Verification items for the finished model (mm, model axes). Round coordinates to 2 decimals unless told otherwise and drop trailing zeros. Order: outer loops, then holes, each group sorted by start corner. A loop starts at its lowest first (then second) coordinate and runs counter-clockwise, first axis right, second up. Notation, with made-up numbers: (7, 4.5) -> (46, 4.5) arc R25 cw to (46, 37.5) -> close; hole circle Ø5 at (32.25, 84). An arc over 180 degrees is marked (long way). Put each result on its own line as item: value.
from build123d import *

# Parameters (mm, degrees)
SKETCH1_W           = 100
SKETCH1_H           = 11.7
BOSS_EXTRUDE1_DEPTH = 2.85
SKETCH2_R           = 1.75
CUT_EXTRUDE3_DEPTH  = 51.421671928
SKETCH3_R           = 2.4
CUT_EXTRUDE4_DEPTH  = 51.662732852


with BuildPart() as part:
    # Sketch1 → Boss-Extrude1 (new body)
    with BuildSketch(Plane(origin=(0, 0, 0), x_dir=(1, 0, 0), z_dir=(0, 1, 0))):
        Rectangle(SKETCH1_W, SKETCH1_H)
    extrude(amount=BOSS_EXTRUDE1_DEPTH)

    # Sketch2 → Cut-Extrude3 (cut, through all)
    with BuildSketch(Plane(origin=(0, 2.85, 0), x_dir=(1, 0, 0), z_dir=(0, 1, 0))):
        with Locations(Location((0, 0, 0), (0, 0, 270))):
            Circle(SKETCH2_R)
    extrude(amount=-CUT_EXTRUDE3_DEPTH, mode=Mode.SUBTRACT)

    # Sketch3 → Cut-Extrude4 (cut, through all)
    with BuildSketch(Plane.XZ.offset(2.85)):
        with Locations(Location((-37.5, 0, 0), (0, 0, 270))):
            Circle(SKETCH3_R)
        with Locations(Location((37.5, 0, 0), (0, 0, 270))):
            Circle(SKETCH3_R)
    extrude(amount=-CUT_EXTRUDE4_DEPTH, mode=Mode.SUBTRACT)


solid = part.part
Item 1: Material ranges on L1, parallel to X at y = 1.7, z = 0; L2, parallel to X at y = 1.9, z = 2; L3, parallel to X at y = 1.55, z = 0.5, recorded low to high. Write a range as [from, to].
Check sheet entries:
L1: x = [-50, -39.9], [-35.1, -1.75], [1.75, 35.1], [39.9, 50]
L2: x = [-50, -38.83], [-36.17, 36.17], [38.83, 50]
L3: x = [-50, -39.85], [-35.15, -1.68], [1.68, 35.15], [39.85, 50]
Item 2: Section check B-B on y = 0.9. Record the boundary of the cut face in (x, z), then the cut area to 3 significant figures.
Check sheet entries:
outline: (-50, -5.85) -> (50, -5.85) -> (50, 5.85) -> (-50, 5.85) -> close; hole circle Ø4.8 at (-37.5, 0); hole circle Ø3.5 at (0, 0); hole circle Ø4.8 at (37.5, 0)
area: 1,120 mm^2
Item 3: Release check for a two-part mould opening along X. For faces 1 (the flat face through (-1, 1, -5.85)), 2 (the flat face through (50, 1, 0)), 3 (the cylindrical face through (-39.843, 1.405, 0.52)), 4 (the cylindrical face through (-1.71, 1.44, -0.38)) record: +X half, -X half, draft (parallel to the pull), parting line (faces both ways), or undercut.
Check sheet entries:
face 1: draft
face 2: +X half
face 3: undercut
face 4: undercut
Item 4: Section check A-A on x = 37.5. Record the boundary of the cut face in (y, z), then the cut area to 3 significant figures.
Check sheet entries:
outline: (0, -5.85) -> (2.85, -5.85) -> (2.85, -2.4) -> (0, -2.4) -> close; (0, 2.4) -> (2.85, 2.4) -> (2.85, 5.85) -> (0, 5.85) -> close
area: 19.7 mm^2
